```python
from build123d import *

# Parameters (mm, degrees)
CROQUIS1_W                                           = 190
CROQUIS1_H                                           = 200
CROQUIS1_R                                           = 5
CROQUIS1_R_2                                         = 40
SALIENTE_EXTRUIR1_DEPTH                              = 20
CROQUIS2_OUTSIDE_W                                   = 247.318
CROQUIS2_OUTSIDE_H                                   = 257.318
CROQUIS2_OUTSIDE_R                                   = 50
CORTAR_EXTRUIR1_DEPTH                                = 5
CHAFL_N1_SIZE                                        = 0.5
CHAFL_N2_SIZE                                        = 5
CORTAR_EXTRUIR2_DEPTH                                = 139.744369255
CORTAR_EXTRUIR2_DEPTH_BACK                           = 139.744369255
CROQUIS3_R                                           = 4.375
REFRENTADO_PARA_TORNILLO_TAP_N_CON_CABEZ_D           = 11
REFRENTADO_PARA_TORNILLO_TAP_N_CON_CABEZ_CBORE_D     = 18
REFRENTADO_PARA_TORNILLO_TAP_N_CON_CABEZ_CBORE_DEPTH = 10
TALADRO_ROSCADO_M10X1_01_D                           = 9


with BuildPart() as part:
    # Croquis1 → Saliente-Extruir1 (new body)
    with BuildSketch(Plane.XY):
        Rectangle(CROQUIS1_W, CROQUIS1_H)
        with Locations((80, 0)):
            Circle(CROQUIS1_R, mode=Mode.SUBTRACT)
        with Locations((40, -69.282032303)):
            Circle(CROQUIS1_R, mode=Mode.SUBTRACT)
        with Locations((-40, -69.282032303)):
            Circle(CROQUIS1_R, mode=Mode.SUBTRACT)
        with Locations((-80, 0)):
            Circle(CROQUIS1_R, mode=Mode.SUBTRACT)
        with Locations((-40, 69.282032303)):
            Circle(CROQUIS1_R, mode=Mode.SUBTRACT)
        with Locations((40, 69.282032303)):
            Circle(CROQUIS1_R, mode=Mode.SUBTRACT)
        with Locations((0, 80)):
            Circle(CROQUIS1_R, mode=Mode.SUBTRACT)
        Circle(CROQUIS1_R_2, mode=Mode.SUBTRACT)
    extrude(amount=SALIENTE_EXTRUIR1_DEPTH)

    # Croquis2 outside → Cortar-Extruir1 (cut)
    with BuildSketch(Plane.XY.offset(20)):
        Rectangle(CROQUIS2_OUTSIDE_W, CROQUIS2_OUTSIDE_H)
        Circle(CROQUIS2_OUTSIDE_R, mode=Mode.SUBTRACT)
    extrude(amount=-CORTAR_EXTRUIR1_DEPTH, mode=Mode.SUBTRACT)

    # Chaflán1
    chafl_n1_edges = [part.edges().sort_by_distance(p)[0] for p in [
        (-50, 0, 20),
    ]]
    chamfer(chafl_n1_edges, length=CHAFL_N1_SIZE)

    # Chaflán2
    chafl_n2_edges = [part.edges().sort_by_distance(p)[0] for p in [
        (95, -100, 7.5),
        (-95, -100, 7.5),
        (-95, 100, 7.5),
        (95, 100, 7.5),
    ]]
    chamfer(chafl_n2_edges, length=CHAFL_N2_SIZE)

    # Croquis3 → Cortar-Extruir2 (cut, two sides: drawn at the far end of the back side and taken through both)
    with BuildSketch(Plane.XY.offset(15).offset(-CORTAR_EXTRUIR2_DEPTH_BACK)):
        with Locations((-80, 80)):
            Circle(CROQUIS3_R)
        with Locations((80, 80)):
            Circle(CROQUIS3_R)
        with Locations((80, -80)):
            Circle(CROQUIS3_R)
        with Locations((-80, -80)):
            Circle(CROQUIS3_R)
    extrude(amount=CORTAR_EXTRUIR2_DEPTH + CORTAR_EXTRUIR2_DEPTH_BACK, mode=Mode.SUBTRACT)

    # Refrentado para tornillo tapón con cabeza de clavija de M101 (through all)
    with Locations(Plane(origin=(40, 69.282032303, 0), x_dir=(-1, 0, 0), z_dir=(0, 0, -1))):
        with Locations((0, 0), (-40, -69.282032303), (120, -69.282032303), (80, -138.564064606), (0, -138.564064606), (80, 0)):
            CounterBoreHole(REFRENTADO_PARA_TORNILLO_TAP_N_CON_CABEZ_D / 2, REFRENTADO_PARA_TORNILLO_TAP_N_CON_CABEZ_CBORE_D / 2, REFRENTADO_PARA_TORNILLO_TAP_N_CON_CABEZ_CBORE_DEPTH)

    # Taladro roscado M10x1.01 (through all)
    with Locations(Plane(origin=(0, 0, 0), x_dir=(-1, 0, 0), z_dir=(0, 0, -1))):
        with Locations((-80, 80), (80, 80), (-80, -80), (80, -80)):
            Hole(TALADRO_ROSCADO_M10X1_01_D / 2)


solid = part.part
```
Read the model definition and answer for the solid it produces. Units are mm, in the model's axes. A direction names the side the tool comes from. Coordinates: 2 decimals unless noted, no trailing zeros. Loops run counter-clockwise (first coordinate to the right, second up) from the corner with the lowest first, then second, coordinate; pieces in that order, holes last. Notation, with made-up numbers: (54, -27) - (99, -27) arc R25 ccw to (99, -3) - close; hole circle Ø5 at (-31, -30.75). An arc over 180 degrees is marked (long way). Answer in a Markdown table with one row per item.
1. Straight lines are drawn through the part: line 1 (X direction, y = -69, z = 10.25); line 2 (X direction, y = 83, z = 8); line 3 (Z direction, x = 49, y = 50). For each, find the intervals that lie inside material, in ascending order.
Conclusion:
| item | result |
|---|---|
| line 1 | x = -95 to -45.49, -34.51 to 34.51, 45.49 to 95 |
| line 2 | x = -95 to -83.35, -76.65 to -4, 4 to 76.65, 83.35 to 95 |
| line 3 | z = 0 to 15 |
2. Find section C-C, the plane x = -55.5. Write down the section's boundary in (y, z), then the cut area to 3 significant figures.
Conclusion:
| item | result |
|---|---|
| outline | (-100, 0) - (100, 0) - (100, 15) - (-100, 15) - close |
| area | 3,000 mm² |
3. Find section D-D, the plane y = 2.5. Count the separate pieces of the cut face and the enclosed holes in it, then the cut area to 3 significant figures.
Conclusion:
| item | result |
|---|---|
| separate pieces | 4 |
| enclosed holes | 0 |
| area | 1,310 mm² |
4. Find section B-B, the plane y = 55. Write down the section's boundary in (x, z), then the cut area to 3 significant figures.
Conclusion:
| item | result |
|---|---|
| outline | (-95, 0) - (95, 0) - (95, 15) - (-95, 15) - close |
| area | 2,850 mm² |
5. Which of the six approach directions +Z, -Z, +X, -X, +Y, -Y give full straight-line access (tool end or side, diameter ignored) to faces 1 (the face through (74.505, 0.242, 12.535)), 2 (the face through (-44, -65, 10))?
Conclusion:
| item | result |
|---|---|
| face 1 | +Z, -Z |
| face 2 | -Z |
6. Find section A-A, the plane x = -80. Write down the section's boundary in (y, z), then the cut area to 4 significant figures.
Conclusion:
| item | result |
|---|---|
| outline | (-100, 0) - (-84.5, 0) - (-84.5, 15) - (-100, 15) - close; (-75.5, 0) - (-9, 0) - (-9, 10) - (-5.5, 10) - (-5.5, 15) - (-75.5, 15) - close; (5.5, 10) - (9, 10) - (9, 0) - (75.5, 0) - (75.5, 15) - (5.5, 15) - close; (84.5, 0) - (100, 0) - (100, 15) - (84.5, 15) - close |
| area | 2,495 mm² |
7. Given pin 1 (17.5 mm diameter, centred on x = 40, y = 69.28, fed in from -Z); pin 2 (9 mm diameter, centred on x = -40, y = -69.28, fed in from -Z); pin 3 (3 mm diameter, centred on x = -16.5, z = 17.5, fed in from -Y); pin 4 (3 mm diameter, centred on x = 43, y = 59, fed in from +Z), each flat-ended and moving along its own axis, determine where each tip first touches the part or whether it passes through.
Conclusion:
| item | result |
|---|---|
| pin 1 | stops at z = 10 |
| pin 2 | passes through |
| pin 3 | stops at y = -47.7 |
| pin 4 | stops at z = 15 |
8. Determine the mould class of faces 3 (the face through (95, -1, 7)), 4 (the face through (-1, -100, 7)), 5 (the face through (41.95, -78.07, 4.93)) for opening direction X: +X half, -X half, draft (parallel to the pull), parting line (faces both ways), or undercut.
Conclusion:
| item | result |
|---|---|
| face 3 | +X half |
| face 4 | draft |
| face 5 | undercut |
